```python
from build123d import *

# Parameters (mm, degrees)
BOSS_EXTRUDE1_DEPTH      = 25
BOSS_EXTRUDE1_DEPTH_BACK = 25
CUT_EXTRUDE1_DEPTH       = 161.078105936
CUT_EXTRUDE1_DEPTH_BACK  = 161.078105936
SKETCH2_W                = 40
SKETCH2_H                = 100
SKETCH3_R                = 17.5
BOSS_EXTRUDE2_DEPTH      = 5
CUT_EXTRUDE2_DEPTH       = 10
FILLET1_R                = 20
FILLET2_R                = 4
FILLET1_OF_MIRROR2_R     = 20
FILLET2_OF_MIRROR2_R     = 4


with BuildPart() as part:
    # Sketch1 → Boss-Extrude1 (new, two sides: drawn at the far end of the back side and taken through both)
    with BuildSketch(Plane(origin=(0, 0, 0), x_dir=(0, 0, -1), z_dir=(1, 0, 0)).offset(-BOSS_EXTRUDE1_DEPTH_BACK)):
        with BuildLine():
            Line((-125, -25), (125, -25))
            ThreePointArc((125, -25), (150, 0), (125, 25))
            Line((125, 25), (-125, 25))
            ThreePointArc((-125, 25), (-150, 0), (-125, -25))
        make_face()
    extrude(amount=BOSS_EXTRUDE1_DEPTH + BOSS_EXTRUDE1_DEPTH_BACK)

    # Sketch2 → Cut-Extrude1 (cut, two sides: drawn at the far end of the back side and taken through both)
    with BuildSketch(Plane(origin=(0, 25, 0), x_dir=(1, 0, 0), z_dir=(0, 1, 0)).offset(-CUT_EXTRUDE1_DEPTH_BACK)):
        with Locations((0, 150)):
            Rectangle(SKETCH2_W, SKETCH2_H)
    extrude(amount=CUT_EXTRUDE1_DEPTH + CUT_EXTRUDE1_DEPTH_BACK, mode=Mode.SUBTRACT)

    # Sketch3 → Boss-Extrude2 (add)
    with BuildSketch(Plane(origin=(25, 0, 0), x_dir=(0, 0, -1), z_dir=(1, 0, 0))):
        with Locations(Location((125, 0, 0), (0, 0, 180))):
            Circle(SKETCH3_R)
    boss_extrude2 = extrude(amount=BOSS_EXTRUDE2_DEPTH)

    # Mirror1: Boss-Extrude2 across plane
    add(boss_extrude2.mirror(Plane(origin=(0, 0, 0), x_dir=(0, 0, 1), z_dir=(1, 0, 0))))

    # Sketch4 → Cut-Extrude2 (cut)
    with BuildSketch(Plane(origin=(25, 0, 0), x_dir=(0, 0, -1), z_dir=(1, 0, 0))):
        with BuildLine():
            Line((-102.639320225, -20), (-5, -20))
            Line((-5, -20), (-74.282032303, 20))
            Line((-74.282032303, 20), (-102.639320225, 20))
            ThreePointArc((-102.639320225, 20), (-96.974829231, 10.704662693), (-95, 0))
            ThreePointArc((-95, 0), (-96.974829231, -10.704662693), (-102.639320225, -20))
        make_face()
        Polygon((0, -17.113248654), (64.282032303, 20), (-64.282032303, 20), align=None)
        with BuildLine():
            ThreePointArc((96.277186767, -20), (90, 0), (96.277186767, 20))
            Line((96.277186767, 20), (74.282032303, 20))
            Line((74.282032303, 20), (5, -20))
            Line((5, -20), (96.277186767, -20))
        make_face()
    cut_extrude2 = extrude(amount=-CUT_EXTRUDE2_DEPTH, mode=Mode.SUBTRACT)

    # Fillet1
    fillet1_edges = [part.edges().sort_by_distance(p)[0] for p in [
        (20, -17.113248654, 0),
        (20, 20, -74.282032303),
        (20, 20, 74.282032303),
    ]]
    fillet(fillet1_edges, radius=FILLET1_R)

    # Fillet2
    fillet2_edges = [part.edges().sort_by_distance(p)[0] for p in [
        (20, 20, 64.282032303),
        (20, 20, -64.282032303),
        (20, 20, -96.277186767),
        (20, -20, -96.277186767),
        (20, -20, -5),
        (20, -20, 102.639320225),
        (20, 20, 102.639320225),
        (20, -20, 5),
    ]]
    fillet(fillet2_edges, radius=FILLET2_R)

    # Mirror2: Cut-Extrude2 across plane
    add(cut_extrude2.mirror(Plane(origin=(0, 0, 0), x_dir=(0, 0, 1), z_dir=(1, 0, 0))), mode=Mode.SUBTRACT)

    # Fillet1 of Mirror2
    fillet1_of_mirror2_edges = [part.edges().sort_by_distance(p)[0] for p in [
        (-20, -17.113248654, 0),
        (-20, 20, -74.282032303),
        (-20, 20, 74.282032303),
    ]]
    fillet(fillet1_of_mirror2_edges, radius=FILLET1_OF_MIRROR2_R)

    # Fillet2 of Mirror2
    fillet2_of_mirror2_edges = [part.edges().sort_by_distance(p)[0] for p in [
        (-20, 20, 64.282032303),
        (-20, 20, -64.282032303),
        (-20, 20, -96.277186767),
        (-20, -20, -96.277186767),
        (-20, -20, -5),
        (-20, -20, 102.639320225),
        (-20, 20, 102.639320225),
        (-20, -20, 5),
    ]]
    fillet(fillet2_of_mirror2_edges, radius=FILLET2_OF_MIRROR2_R)


solid = part.part
```
The model under review builds one solid part; all positions refer to its coordinate system, in mm. A direction names the side the tool comes from. Coordinates: 2 decimals unless noted, no trailing zeros. Write each loop counter-clockwise with the first axis right and the second up, starting at its lowest first coordinate (ties: lowest second). Pieces come first, ordered by that corner, then holes. Notation, with made-up numbers: (80, -38) - (112, -38) arc R18 ccw to (112, -30) - close; hole circle Ø2 at (8, 54.25). An arc over 180 degrees is marked (long way). Write item = value, one per line.
(1) Consider section C-C, the plane z = 60. Give the boundary of the cut face in (x, y).
Result sheet:
outline = (-25, -25) - (25, -25) - (25, -20) - (15, -20) - (15, 11.75) - (25, 11.75) - (25, 25) - (-25, 25) - (-25, 11.75) - (-15, 11.75) - (-15, -20) - (-25, -20) - close
(2) Consider section B-B, the plane x = -1.5. Give the boundary of the cut face in (y, z), then the cut area to 3 significant figures.
Result sheet:
outline = (-25, -100) - (25, -100) - (25, 125) arc R25 ccw to (-25, 125) - close
area = 12,200 mm^2
(3) For P1, Ø10, axis at y = 19.5, z = 50, coming from the +X side; P2, Ø12, axis at y = 15.5, z = -95, coming from the -X side; P3, Ø4, axis at x = 5, y = -16, coming from the -Z side, all flat-tipped, find the tip position at first contact; note any pin that passes through.
Result sheet:
P1 = 25
P2 = -25
P3 = -100
(4) For line 1 (Y direction, x = 19.5, z = -34); line 2 (X direction, y = -15.5, z = -133); line 3 (Z direction, x = -23, y = -9.5), list the stretches that pass through material, from the lowest coordinate up. Write a range as [from, to].
Result sheet:
line_1 = [-25, -20], [-3.26, 2.52], [20, 25]
line_2 = [-30, -20], [20, 30]
line_3 = [-148.12, -91.31], [-23.19, -13.19], [13.19, 23.19], [96.54, 148.12]
(5) Consider section A-A, the plane z = -57. Give the boundary of the cut face in (x, y), then the cut area to 3 significant figures.
Result sheet:
outline = (-25, -25) - (25, -25) - (25, -20) - (15, -20) - (15, 10.02) - (25, 10.02) - (25, 25) - (-25, 25) - (-25, 10.02) - (-15, 10.02) - (-15, -20) - (-25, -20) - close
area = 1,900 mm^2
(6) Machinability: for faces 1 (the face through (-27.465, 6.703, -108.834)), 2 (the face through (0, 25, -2)), 3 (the face through (20, 20, -85)), which of the approach directions +Z, -Z, +X, -X, +Y, -Y give a long, thin tool a straight path to every point of the face, cutting with its end or side? Answer none if there is none.
Result sheet:
face_1 = -X
face_2 = +Z, -Z, +X, -X, +Y
face_3 = +X
(7) Mouldability with a two-part tool opening along Y and no side actions: class faces 4 (the face through (20, 0, -125)), 5 (the face through (22.465, -0.55, -149.994)), 6 (the face through (-19.93, -16.964, 16.046)), 7 (the face through (-20, 20, -1)) as pulls with the +Y half, pulls with the -Y half, needs draft (parallel to the pull), parting line crosses it, or undercut.
Result sheet:
face_4 = needs draft
face_5 = parting line crosses it
face_6 = undercut
face_7 = undercut
